Solid Edge part; units mm, degrees
sketch "Sketch1" plane through (0, 0, 0) normal (0, -1, 0) x (1, 0, 0)
  line L0 (0, 0) -> (3.4, 0)
  arc A0 (3.4, 0) -> (4.25, -0.85) centre (3.4, -0.85) cw
  line L1 (4.25, -0.85) -> (4.25, -5)
  line L2 (4.25, -5) -> (2.5, -5)
  line L3 (2.5, -5) -> (2.5, -54.2)
  line L4 (2.5, -54.2) -> (1.7, -55)
  line L5 (1.7, -55) -> (0, -55)
revolve "RevolvedProtrusion1" add sketch "Sketch1" angle 360 about axis through (0, 0, -55) along (0, 0, 1)
sketch "Sketch2" plane through (0, 0, 0) normal (0, 0, 1) x (1, 0, 0)
  line L0 (-2, -1.1547) -> (-2, 1.1547)
  line L1 (-2, 1.1547) -> (0, 2.3094)
  line L2 (0, 2.3094) -> (2, 1.1547)
  line L3 (2, 1.1547) -> (2, -1.1547)
  line L4 (2, -1.1547) -> (0, -2.3094)
  line L5 (0, -2.3094) -> (-2, -1.1547)
extrude "Cutout1" cut sketch "Sketch2" against normal blind 2.5
sketch "Sketch3" plane through (0, 0, 0) normal (1, 0, 0) x (0, 1, 0)
  line L0 (0, -3.8333) -> (2.3094, -2.5)
  line L1 (0, -2.5) -> (2.3094, -2.5)
  line L2 (0, -2.5) -> (0, -3.8333)
revolve "RevolvedCutout1" cut sketch "Sketch3" angle 360 about axis through (0, 0, -60.325) along (0, 0, 1)
cosmetic_thread "Thread1"
The model under review builds one solid part; all positions refer to its coordinate system, in mm. A direction names the side the tool comes from. Give positions to 0.01 mm unless a question says otherwise; leave off trailing zeros. Write each loop counter-clockwise with the first axis right and the second up, starting at its lowest first coordinate (ties: lowest second). Pieces come first, ordered by that corner, then holes. Notation, with made-up numbers: M 76,29.5 L 93,29.5 A35 ccw 93,64.5 Z; hole C -9.75,-32 d5. An arc over 180 degrees is marked long. Write item = value, one per line. Start each with the question number.
Q1. For line 1 (X direction, y = -1.5, z = -27.5); line 2 (Z direction, x = -2.5, y = 1), list the stretches that pass through material, from the lowest coordinate up.
Q2. We need section A-A (z = -16.5). State the section outline as (x, y) points, plus the area to 3 significant figures.
Q3. Machinability: for faces 1 (the face through (0, 0, -55)), 2 (the face through (-0.99, -1.74, -1.23)), 3 (the face through (-0.54, 2.44, -29.94)), which of the approach directions +Z, -Z, +X, -X, +Y, -Y give a long, thin tool a straight path to every point of the face, cutting with its end or side? Answer none if there is none.
Q4. Mouldability with a two-part tool opening along X and no side actions: class faces 4 (the face through (2.285, -3.584, -2.954)), 5 (the face through (0.39, -0.09, -3.6)), 6 (the face through (2, -2, -5)) as released by +X, released by -X, zero draft, split by the parting line, or undercut.
Q5. Clearance check with flat-ended pins moving along their axes: pin 1 (2 mm diameter, centred on x = -3, y = 1.5, fed in from -Z); pin 2 (1.3 mm diameter, centred on x = -1.5, y = -2, fed in from -Z); pin 3 (1 mm diameter, centred on y = 1.5, z = -13, fed in from -X). State where each tip first meets the part, or that it passes through.
Result set:
q1.line_1 = -2 to 2
q1.line_2 = -5 to 0
q2.outline = C 0,0 d5
q2.area = 19.6 mm2
q3.face_1 = -Z, +X, -X, +Y, -Y
q3.face_2 = +Z
q3.face_3 = -Z
q4.face_4 = split by the parting line
q4.face_5 = undercut
q4.face_6 = zero draft
q5.pin_1 = -54.35
q5.pin_2 = -54.85
q5.pin_3 = -2.29
